Input: dimensioned drawing with shaded views. Units: mm. Origin: part minimum x, y, z. Round coordinates to 2 decimals unless told otherwise and drop trailing zeros. Loops run counter-clockwise (first coordinate to the right, second up) from the corner with the lowest first, then second, coordinate; pieces in that order, holes last. Notation, with made-up numbers: M 72.5,33.25 L 127.5,33.25 A36 cw 127.5,71.25 Z; hole C 83.5,40 d11. An arc over 180 degrees is marked long. Answer as CSV lines item,"result". Start each with the question number.
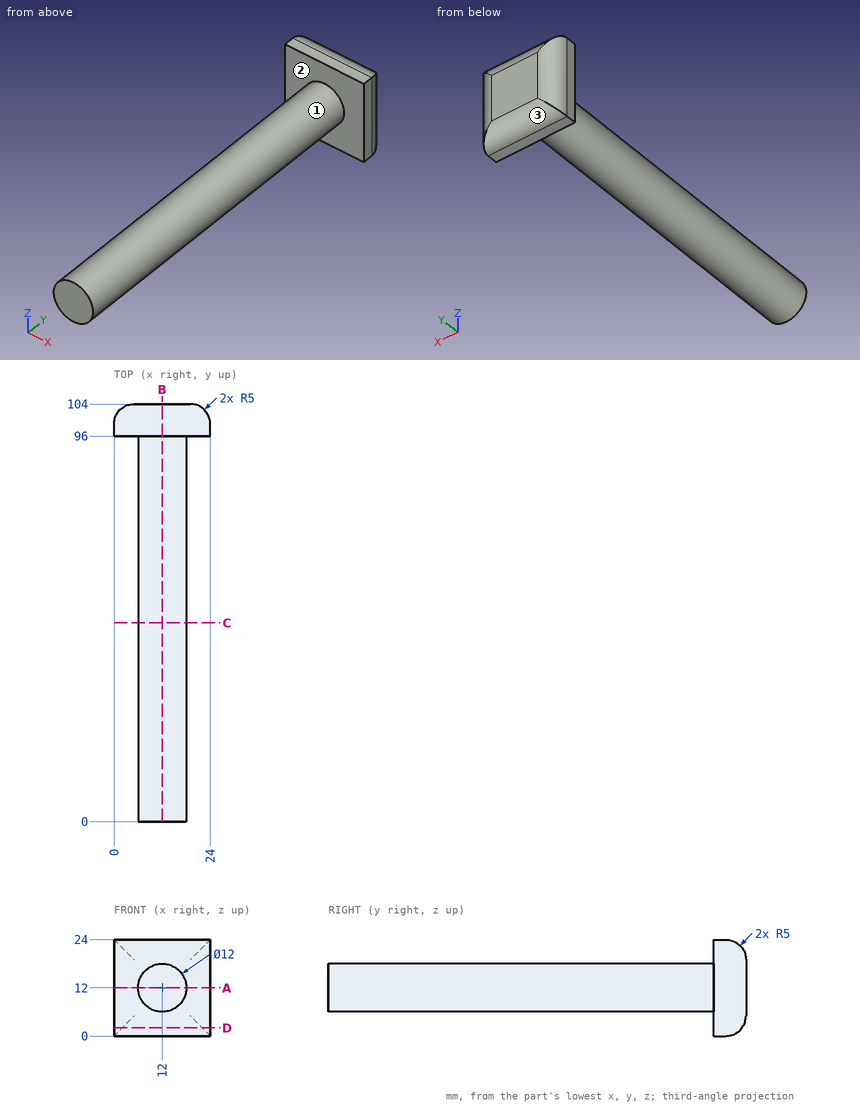
1) Contact query for flat-ended pins moving along their axis: pin 1 Ø12 at (y, z) = (28, 9) entering from +X; pin 2 Ø8 at (x, y) = (16.5, 25) entering from +Z; pin 3 Ø6 at (x, y) = (5, 76) entering from -Z; pin 4 Ø12 at (x, z) = (8.5, 13.5) entering from -Y. Output: stop coordinate, or through.
2) Mould query, pull axis Z, two halves, no side actions, for the marked faces 1, 2 and 3. Classes: pulls with the +Z half, pulls with the -Z half, needs draft (parallel to the pull), parting line crosses it, or undercut.
3) Section B-B, the plane x = 12. Return loops of the section in (y, z), and give its area (3 significant figures).
4) Section A-A, the plane z = 12. Return loops of the section in (x, y), and give its area (3 significant figures).
5) Section D-D, the plane z = 2. Return loops of the section in (x, y), and give its area (3 significant figures).
6) Ray query, line 1 along X through (y, z) = (61, 11.5); line 2 along Y through (x, z) = (7.5, 7.5); line 3 along X through (y, z) = (83, 16). Return the intervals inside material, ascending.
7) Section C-C, the plane y = 49.5. Return loops of the section in (x, z).
Findings below:
1,pin 1,"x = 18"
1,pin 2,"z = 17.98"
1,pin 3,"z = 7.53"
1,pin 4,"y = 0"
2,face 1,"parting line crosses it"
2,face 2,"needs draft"
2,face 3,"pulls with the -Z half"
3,outline,"M 0,6 L 96,6 L 96,0 L 99,0 A5 ccw 104,5 L 104,19 A5 ccw 99,24 L 96,24 L 96,18 L 0,18 Z"
3,area,"1,330 mm²"
4,outline,"M 0,96 L 6,96 L 6,0 L 18,0 L 18,96 L 24,96 L 24,99 A5 ccw 19,104 L 5,104 A5 ccw 0,99 Z"
4,area,"1,330 mm²"
5,outline,"M 0,96 L 24,96 L 24,99 A5 ccw 22,103 L 2,103 A5 ccw 0,99 Z"
5,area,"163 mm²"
6,line 1,"6.02 to 17.98"
6,line 2,"96 to 104"
6,line 3,"7.53 to 16.47"
7,outline,"C 12,12 d12"
